from build123d import *

# Parameters (mm, degrees)
SKETCH2_R           = 28
BOSS_EXTRUDE1_DEPTH = 5
SKETCH3_W           = 5
SKETCH3_H           = 20
CUT_EXTRUDE1_DEPTH  = 10


with BuildPart() as part:
    # Sketch1 → Revolve1 (revolve)
    with BuildSketch(Plane.XY):
        with BuildLine():
            Line((-24.662024669, 18.27739706), (-24.662024669, -43.219960911))
            Line((-24.662024669, -43.219960911), (0, -43.219960911))
            Line((0, -43.219960911), (0, 42.939421729))
            ThreePointArc((0, 42.939421729), (-17.438684882, 35.716081941), (-24.662024669, 18.27739706))
        make_face()
    revolve(axis=Axis((0, -43.219960911, 0), (0, 1, 0)))

    # Sketch2 → Boss-Extrude1 (add)
    with BuildSketch(Plane.XZ.offset(43.219960911)):
        with Locations(Location((0, 0, 0), (0, 0, 270))):
            Circle(SKETCH2_R)
    extrude(amount=BOSS_EXTRUDE1_DEPTH)

    # Sketch3 → Cut-Extrude1 (cut)
    with BuildSketch(Plane.XZ.offset(48.219960911)):
        Rectangle(SKETCH3_W, SKETCH3_H)
    extrude(amount=-CUT_EXTRUDE1_DEPTH, mode=Mode.SUBTRACT)


solid = part.part
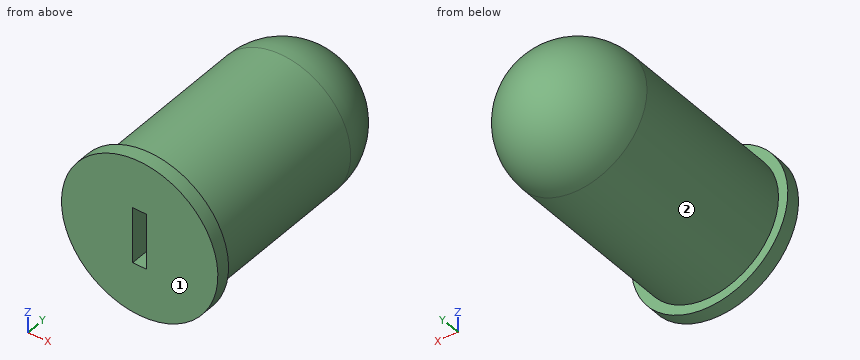
Can you work these out from the model? Positions are in its coordinate system, mm. Face numbers are marked on the shaded views. A direction names the side the tool comes from. Round coordinates to 2 decimals unless told otherwise and drop trailing zeros. Loops run counter-clockwise (first coordinate to the right, second up) from the corner with the lowest first, then second, coordinate; pieces in that order, holes last. Notation, with made-up numbers: (86.25, 67) - (115.25, 67) arc R18 ccw to (115.25, 92) - close; hole circle Ø1 at (-34, 51.25). An arc over 180 degrees is marked (long way). Write item = value, one per line. Start each with the question number.
(1) For P1, Ø1.5, axis at x = -1, z = -2, coming from the -Y side; P2, Ø8, axis at x = 9.5, y = -24.5, coming from the -Z side; P3, Ø5, axis at y = -43, z = 0, coming from the +X side, each with a flat end and sliding along its axis, tell me the tip position at first contact or that it passes through.
(2) If we section it at C-C (y = 11): Please give me the cut outline in (x, z), and give its area (3 significant figures).
(3) If we section it at B-B (x = 9): Please give me the cut outline in (y, z), and give its area (3 significant figures).
(4) If I drill on probe 1 along Y at (x, z) = (1.5, 26); probe 2 along X at (y, z) = (14.5, 1); probe 3 along X at (y, z) = (-38.5, 5.5), over which ranges is the centre line in solid material (lowest first)? Write a range as [from, to].
(5) If we section it at D-D (x = 0): Please give me the cut outline in (y, z).
(6) If we section it at A-A (z = 0): Please give me the cut outline in (x, y), and give its area (3 significant figures).
(7) For the marked faces 1 and 2, which set-ups out of +Z, -Z, +X, -X, +Y, -Y let a thin tool reach every point of the face, with its end or its side?
Ans:
q1.P1 = -38.22
q1.P2 = -24.04
q1.P3 = 28
q2.outline = circle Ø49.32 at (0, 0)
q2.area = 1,910 mm²
q3.outline = (-48.22, -26.51) - (-43.22, -26.51) - (-43.22, -22.96) - (18.28, -22.96) arc R22.96 ccw to (18.28, 22.96) - (-43.22, 22.96) - (-43.22, 26.51) - (-48.22, 26.51) - close
q3.area = 3,920 mm²
q4.probe_1 = [-48.22, -43.22]
q4.probe_2 = [-24.64, 24.64]
q4.probe_3 = [-24.04, -2.5], [2.5, 24.04]
q5.outline = (-48.22, -28) - (-43.22, -28) - (-43.22, -24.66) - (18.28, -24.66) arc R24.66 ccw to (18.28, 24.66) - (-43.22, 24.66) - (-43.22, 28) - (-48.22, 28) - (-48.22, 10) - (-38.22, 10) - (-38.22, -10) - (-48.22, -10) - close
q6.outline = (-28, -48.22) - (-2.5, -48.22) - (-2.5, -38.22) - (2.5, -38.22) - (2.5, -48.22) - (28, -48.22) - (28, -43.22) - (24.66, -43.22) - (24.66, 18.28) arc R24.66 ccw to (-24.66, 18.28) - (-24.66, -43.22) - (-28, -43.22) - close
q6.area = 4,220 mm²
q7.face_1 = +Z, -Z, +X, -X, -Y
q7.face_2 = +Y
